Source: CAD feature listing. Evaluate the final solid. Frame: model axes, mm. A direction names the side the tool comes from. Coordinates: 2 decimals unless noted, no trailing zeros. Loops run counter-clockwise (first coordinate to the right, second up) from the corner with the lowest first, then second, coordinate; pieces in that order, holes last. Notation, with made-up numbers: (46.5, 17) -> (60.5, 17) arc R20 ccw to (60.5, 28) -> close; hole circle Ø9 at (10, 29). An arc over 180 degrees is marked (long way). Answer as CSV lines item,"result".
from build123d import *

# Parameters (mm, degrees)
F0_W     = 42
F0_H     = 42
F1_DEPTH = 48
F2_R     = 1.5
F3_DEPTH = 10
F2_R_2   = 11
F4_DEPTH = 2
F5_R     = 2.5
F6_DEPTH = 22
F8_DEPTH = 15
F9_SIZE  = 3


with BuildPart() as f1:
    # F0 (on Top) → F1 (new body)
    with BuildSketch(Plane.XY):
        Rectangle(F0_W, F0_H)
    extrude(amount=F1_DEPTH)

    # F2 (on face) → F3 (cut)
    with BuildSketch(Plane.XY.offset(48)):
        with Locations((-15.5, -15.5)):
            Circle(F2_R)
        with Locations((-15.5, 15.5)):
            Circle(F2_R)
        with Locations((15.5, 15.5)):
            Circle(F2_R)
        with Locations((15.5, -15.5)):
            Circle(F2_R)
    extrude(amount=-F3_DEPTH, mode=Mode.SUBTRACT)

    # F2 (on face) → F4 (join)
    with BuildSketch(Plane.XY.offset(48)):
        Circle(F2_R_2)
    extrude(amount=F4_DEPTH)

    # F5 (on face) → F6 (join)
    with BuildSketch(Plane.XY.offset(50)):
        Circle(F5_R)
    extrude(amount=F6_DEPTH)

    # F7 (on face) → F8 (cut)
    with BuildSketch(Plane.XY.offset(72)):
        with BuildLine():
            ThreePointArc((1.5, 2), (0, 2.5), (-1.5, 2))
            Line((-1.5, 2), (1.5, 2))
        make_face()
    extrude(amount=-F8_DEPTH, mode=Mode.SUBTRACT)

    # F9
    f9_edges = [f1.edges().sort_by_distance(p)[0] for p in [
        (21, -21, 24),
        (21, 21, 24),
        (-21, -21, 24),
        (-21, 21, 24),
    ]]
    chamfer(f9_edges, length=F9_SIZE)


solid = f1.part
(1) Cut plane B-B (y = -15.5). Return the cut outline in (x, z).
Computed values:
outline,"(-21, 0) -> (21, 0) -> (21, 48) -> (17, 48) -> (17, 38) -> (14, 38) -> (14, 48) -> (-14, 48) -> (-14, 38) -> (-17, 38) -> (-17, 48) -> (-21, 48) -> close"
(2) Access query for faces 1 (the flat face through (-19, -20, 24)), 2 (the cylindrical face through (14, -15.43, 43.07)). Directions: +Z, -Z, +X, -X, +Y, -Y. A direction counts if a zero-diameter tool reaches every point of the face in a straight line with its end or side. Return the directions, or none.
Computed values:
face 1,"+Z, -Z, -X, -Y"
face 2,"+Z"
(3) Draft query along Y for faces 3 (the cylindrical face through (-17, -15.43, 43.07)), 4 (the flat face through (20, 19, 24)), 5 (the cylindrical face through (-0.54, -2.44, 60.85)). Return one class per face: released by +Y, released by -Y, zero draft, split by the parting line, or undercut.
Computed values:
face 3,"undercut"
face 4,"released by +Y"
face 5,"split by the parting line"
(4) Material intervals for L1, parallel to Y at x = -15.5, z = 41.25; L2, parallel to X at y = -15, z = 42; L3, parallel to Z at x = 12, y = -18, sorted ascending. Write a range as [from, to].
Computed values:
L1,"[-21, -17], [-14, 14], [17, 21]"
L2,"[-21, -16.91], [-14.09, 14.09], [16.91, 21]"
L3,"[0, 48]"
(5) Cut plane C-C (x = 0). Return the cut outline in (y, z), then the cut area to 3 significant figures.
Computed values:
outline,"(-21, 0) -> (21, 0) -> (21, 48) -> (11, 48) -> (11, 50) -> (2.5, 50) -> (2.5, 57) -> (2, 57) -> (2, 72) -> (-2.5, 72) -> (-2.5, 50) -> (-11, 50) -> (-11, 48) -> (-21, 48) -> close"
area,"2,160 mm^2"
(6) Cut plane D-D (z = 54). Return the cut outline in (x, y), then the cut area to 3 significant figures.
Computed values:
outline,"circle Ø5 at (0, 0)"
area,"19.6 mm^2"
(7) Pin query (flat end, axial travel): pin 1 Ø1.5 at (x, y) = (16, -15) entering from +Z; pin 2 Ø2.5 at (x, y) = (-15.5, 16) entering from +Z; pin 3 Ø3.5 at (x, z) = (0, 68) entering from +Y. Return the tip coordinate at first contact, or that it passes through.
Computed values:
pin 1,"z = 38"
pin 2,"z = 48"
pin 3,"y = 2"
(8) Cut plane A-A (z = 40). Return the cut outline in (x, y), then the cut area to 3 significant figures.
Computed values:
outline,"(-21, -18) -> (-18, -21) -> (18, -21) -> (21, -18) -> (21, 18) -> (18, 21) -> (-18, 21) -> (-21, 18) -> close; hole circle Ø3 at (-15.5, -15.5); hole circle Ø3 at (-15.5, 15.5); hole circle Ø3 at (15.5, -15.5); hole circle Ø3 at (15.5, 15.5)"
area,"1,720 mm^2"
